Geometry check sheet. Reference: the model listing, model coordinates, mm. A direction names the side the tool comes from. Round coordinates to 2 decimals unless told otherwise and drop trailing zeros. Loops run counter-clockwise (first coordinate to the right, second up) from the corner with the lowest first, then second, coordinate; pieces in that order, holes last. Notation, with made-up numbers: M 89.5,65.25 L 140.5,65.25 A22 cw 140.5,80.25 Z; hole C 1.5,-24 d3. An arc over 180 degrees is marked long. Write item = value, one per line.
from build123d import *

# Parameters (mm, degrees)
CROQUIS1_R              = 23
CROQUIS1_R_2            = 3.5
SALIENTE_EXTRUIR1_DEPTH = 3


with BuildPart() as part:
    # Croquis1 → Saliente-Extruir1 (new body)
    with BuildSketch(Plane(origin=(0, 0, 0), x_dir=(1, 0, 0), z_dir=(0, 1, 0))):
        with Locations(Location((0, 0, 0), (0, 0, 270))):
            Circle(CROQUIS1_R)
        with BuildLine():
            Line((1.5, 2), (1.5, -2))
            ThreePointArc((1.5, -2), (0, -2.5), (-1.5, -2))
            Line((-1.5, -2), (-1.5, 2))
            ThreePointArc((-1.5, 2), (0, 2.5), (1.5, 2))
        make_face(mode=Mode.SUBTRACT)
        with Locations(Location((18.5, 0, 0), (0, 0, 270))):
            Circle(CROQUIS1_R_2, mode=Mode.SUBTRACT)
    extrude(amount=SALIENTE_EXTRUIR1_DEPTH)


solid = part.part
(1) Sectioned sample at B-B on y = 1.6. Record the cut outline in (x, z).
Result set:
outline = C 0,0 d46; hole M -1.5,-2 A2.5 ccw 1.5,-2 L 1.5,2 A2.5 ccw -1.5,2 Z; hole C 18.5,0 d7
(2) Sectioned sample at C-C on x = 11. Record the cut outline in (y, z).
Result set:
outline = M 0,-20.2 L 3,-20.2 L 3,20.2 L 0,20.2 Z
(3) Sectioned sample at A-A on z = 0. Record the cut outline in (x, y), then the cut area to 3 significant figures.
Result set:
outline = M -23,0 L -1.5,0 L -1.5,3 L -23,3 Z; M 1.5,0 L 15,0 L 15,3 L 1.5,3 Z; M 22,0 L 23,0 L 23,3 L 22,3 Z
area = 108 mm2
(4) Tool access check on faces 4 (the flat face through (-5, 0, 0)), 5 (the flat face through (-1.5, 1, 0)). Record the directions out of +Z, -Z, +X, -X, +Y, -Y that give a thin tool (end or side, any length) a straight path to the whole face; none if there is none.
Result set:
face_4 = +Z, -Z, +X, -X, -Y
face_5 = +Y, -Y
(5) Sectioned sample at D-D on z = -12. Record the cut outline in (x, y), then the cut area to 3 significant figures.
Result set:
outline = M -19.62,0 L 19.62,0 L 19.62,3 L -19.62,3 Z
area = 118 mm2
(6) Release check for a two-part mould opening along X. For faces 1 (the cylindrical face through (19.394, 1.479, 12.365)), 2 (the flat face through (-5, 3, 0)), 3 (the cylindrical face through (0, 1.5, -2.5)) record: released by +X, released by -X, zero draft, split by the parting line, or undercut.
Result set:
face_1 = split by the parting line
face_2 = zero draft
face_3 = undercut
(7) Depth check by flat-ended pin: pin 1 Ø12 at (x, z) = (-15.5, 0.5) entering from -Y; pin 2 Ø1.5 at (x, y) = (6, 0.5) entering from +Z; pin 3 Ø1.5 at (y, z) = (1.5, 0.5) entering from -X; pin 4 Ø1 at (x, y) = (15, 2) entering from -Z. Enter the tip coordinate at first touch or a pass-through.
Result set:
pin_1 = 0
pin_2 = 22.39
pin_3 = -23
pin_4 = -17.85
(8) Material ranges on line 1 along X through (y, z) = (0.6, 0); line 2 along X through (y, z) = (2.9, 1.5); line 3 along Z through (x, y) = (-1, 2.8), recorded low to high. Write a range as from..to.
Result set:
line_1 = -23..-1.5, 1.5..15, 22..23
line_2 = -22.95..-1.5, 1.5..15.34, 21.66..22.95
line_3 = -22.98..-2.29, 2.29..22.98
